```python
from build123d import *
from build123d.topology import SkipClean

# Parameters (mm, degrees)
SKETCH1_R                      = 2.38125
BOSS_EXTRUDE1_DEPTH            = 11.1125
F_8_32_TAPPED_HOLE1_AT_2_COUNT = 2
F_8_32_TAPPED_HOLE1_AT_2_PITCH = 12.857770024
F_8_32_TAPPED_HOLE1_AT_3_COUNT = 2
F_8_32_TAPPED_HOLE1_AT_3_PITCH = 12.857770024


with BuildPart() as part:
    # Sketch1 → Boss-Extrude1 (new body)
    with BuildSketch(Plane.XY):
        with BuildLine():
            ThreePointArc((0, -6.35), (-6.35, 0), (0, 6.35))
            Line((0, 6.35), (0, 10.795))
            ThreePointArc((0, 10.795), (-2.197021558, 10.569064352), (-4.302077301, 9.900714918))
            ThreePointArc((-4.302077301, 9.900714918), (-9.054681629, 9.776106511), (-12.561760448, 12.985962165))
            ThreePointArc((-12.561760448, 12.985962165), (-19.192123591, 15.444267147), (-21.855781895, 8.89370204))
            ThreePointArc((-21.855781895, 8.89370204), (-21.424604414, 5.897029127), (-22.429987657, 3.041303808))
            ThreePointArc((-22.429987657, 3.041303808), (-23.33625, 0), (-22.429987657, -3.041303808))
            ThreePointArc((-22.429987657, -3.041303808), (-21.424604414, -5.897029127), (-21.855781895, -8.89370204))
            ThreePointArc((-21.855781895, -8.89370204), (-19.192123591, -15.444267147), (-12.561760448, -12.985962165))
            ThreePointArc((-12.561760448, -12.985962165), (-9.054681629, -9.776106511), (-4.302077301, -9.900714918))
            ThreePointArc((-4.302077301, -9.900714918), (-2.197021558, -10.569064352), (0, -10.795))
            Line((0, -10.795), (0, -6.35))
        make_face()
        with Locations((-17.78, 0)):
            Circle(SKETCH1_R, mode=Mode.SUBTRACT)
    extrude(amount=BOSS_EXTRUDE1_DEPTH)

    # Sketch2 → #8-32 Tapped Hole1 (revolve, cut)
    with BuildSketch(Plane(origin=(-10.16, 0, 11.1125), x_dir=(0, -1, 0), z_dir=(1, 0, 0))):
        Polygon((0, 0), (0, 11.1125), (2.72923, 11.1125), (1.7272, 9.959796345), (1.7272, 1.139554944), (2.7178, 0), align=None)
    f_8_32_tapped_hole1 = revolve(axis=Axis((-10.16, 0, 17.4625), (0, 0, -1)), mode=Mode.SUBTRACT)

    # #8-32 Tapped Hole1 at 2: #8-32 Tapped Hole1 ×2
    with Locations(*[Vector(-0.5432512781572743, 0.8395701571521511, 0) * (i * F_8_32_TAPPED_HOLE1_AT_2_PITCH) for i in range(1, F_8_32_TAPPED_HOLE1_AT_2_COUNT)]):
        add(f_8_32_tapped_hole1, mode=Mode.SUBTRACT)

    # #8-32 Tapped Hole1 at 3: #8-32 Tapped Hole1 ×2
    with Locations(*[Vector(-0.5432512781572741, -0.8395701571521512, 0) * (i * F_8_32_TAPPED_HOLE1_AT_3_PITCH) for i in range(1, F_8_32_TAPPED_HOLE1_AT_3_COUNT)]):
        add(f_8_32_tapped_hole1, mode=Mode.SUBTRACT)

    # Mirror2: part across plane


with BuildPart() as part_1:
    with SkipClean():  # the faces are left unmerged after this step: merging them gives an invalid solid
        add(part.part)
        add(part.part.mirror(Plane(origin=(0, 6.35, 11.1125), x_dir=(0, 0, 1), z_dir=(-1, 0, 0))))


solid = part_1.part
```
The model under review builds one solid part; all positions refer to its coordinate system, in mm. Round coordinates to 2 decimals unless told otherwise and drop trailing zeros. Order: outer loops, then holes, each group sorted by start corner. A loop starts at its lowest first (then second) coordinate and runs counter-clockwise, first axis right, second up. Notation, with made-up numbers: (12, 73.25) -> (69, 73.25) arc R26 ccw to (69, 89.25) -> close; hole circle Ø2 at (-6.5, -13). An arc over 180 degrees is marked (long way). One line per item, written item: value. Start each with the question number.
Q1. Clearance check with flat-ended pins moving along their axes: pin 1 Ø5 at (y, z) = (7, 3) entering from -X; pin 2 Ø1.5 at (x, z) = (-4, 10) entering from +Y; pin 3 Ø4 at (x, y) = (-10.16, 0) entering from -Z. State where each tip first meets the part, or that it passes through.
Q2. Mouldability with a two-part tool opening along Y and no side actions: class faces 1 (the face through (1.907, -6.057, 5.478)), 2 (the face through (9.12, -9.8, 5.48)), 3 (the face through (23.336, 0.045, 5.478)), 4 (the face through (21.43, -5.85, 5.48)) as released by +Y, released by -Y, zero draft, split by the parting line, or undercut.
Q3. Take a section at C-C (y = 4.5). Write out the cut boundary in (x, z), and give its area (3 significant figures).
Q4. Take a section at B-B (x = -10.16). Write out the cut boundary in (y, z).
Q5. Take a section at A-A (y = 0). Count the separate pieces of the cut face and the enclosed holes in it, and give its area (3 significant figures).
Q6. Wall thickness on line 1 (X direction, y = -1.5, z = 3); line 2 (X direction, y = 0.5, z = 2); line 3 (X direction, y = 12, z = 5.75): over which ranges is each line inside the solid? List them lowest first.
Reported:
1. pin 1: stops at x = -22.06
1. pin 2: stops at y = 10.29
1. pin 3: stops at z = 0.84
2. face 1: undercut
2. face 2: released by -Y
2. face 3: split by the parting line
2. face 4: undercut
3. outline: (-21.72, 0) -> (-4.48, 0) -> (-4.48, 11.11) -> (-21.72, 11.11) -> close; (4.48, 0) -> (21.72, 0) -> (21.72, 11.11) -> (4.48, 11.11) -> close
3. area: 383 mm2
4. outline: (-10.32, 0) -> (-2.73, 0) -> (-1.73, 1.15) -> (-1.73, 9.97) -> (-2.72, 11.11) -> (-10.32, 11.11) -> close; (1.73, 1.15) -> (2.73, 0) -> (10.32, 0) -> (10.32, 11.11) -> (2.72, 11.11) -> (1.73, 9.97) -> close
5. separate pieces: 6
5. enclosed holes: 0
5. area: 190 mm2
6. line 1: x = -23.13 to -19.63, -15.93 to -11.02, -9.3 to -6.17, 6.17 to 9.3, 11.02 to 15.93, 19.63 to 23.13
6. line 2: x = -23.31 to -20.11, -15.45 to -11.81, -8.51 to -6.33, 6.33 to 8.51, 11.81 to 15.45, 20.11 to 23.31
6. line 3: x = -22.08 to -18.38, -15.91 to -11.98, 11.98 to 15.91, 18.38 to 22.08
